from build123d import *

# Parameters (mm, degrees)
SKETCH1_W           = 50
SKETCH1_H           = 40
SKETCH1_R           = 1.5
SKETCH1_R_2         = 0.75
SKETCH1_R_3         = 2.5
BOSS_EXTRUDE1_DEPTH = 2
FILLET1_R           = 0.3
BOSS_EXTRUDE2_START = 1
SKETCH2_R           = 0.65
BOSS_EXTRUDE2_DEPTH = 2.5
FILLET2_R           = 0.1


with BuildPart() as part:
    # Sketch1 → Boss-Extrude1 (new body)
    with BuildSketch(Plane.XY):
        Rectangle(SKETCH1_W, SKETCH1_H)
        with Locations((-23, 18)):
            Circle(SKETCH1_R, mode=Mode.SUBTRACT)
        with Locations((23, -18)):
            Circle(SKETCH1_R, mode=Mode.SUBTRACT)
        with Locations((8, 8)):
            Circle(SKETCH1_R_2, mode=Mode.SUBTRACT)
        with Locations((-8, -8)):
            Circle(SKETCH1_R_2, mode=Mode.SUBTRACT)
        with Locations((-21, -16)):
            Circle(SKETCH1_R_3, mode=Mode.SUBTRACT)
        with Locations((21, 16)):
            Circle(SKETCH1_R_3, mode=Mode.SUBTRACT)
    extrude(amount=BOSS_EXTRUDE1_DEPTH)

    # Fillet1
    fillet1_edges = [part.edges().sort_by_distance(p)[0] for p in [
        (-25, 0, 2),
        (0, -20, 2),
        (25, 0, 2),
        (0, 20, 2),
    ]]
    fillet(fillet1_edges, radius=FILLET1_R)

    # Sketch2 → Boss-Extrude2 (add)
    with BuildSketch(Plane.XY.offset(BOSS_EXTRUDE2_START)):
        with Locations((-8, 8)):
            Circle(SKETCH2_R)
        with Locations((8, -8)):
            Circle(SKETCH2_R)
    extrude(amount=BOSS_EXTRUDE2_DEPTH)

    # Fillet2
    fillet2_edges = [part.edges().sort_by_distance(p)[0] for p in [
        (-8.65, 8, 2),
        (-8.65, 8, 3.5),
        (7.35, -8, 2),
        (7.35, -8, 3.5),
    ]]
    fillet(fillet2_edges, radius=FILLET2_R)


solid = part.part
Geometry: final body of the model. Coordinates: model frame, mm. A direction names the side the tool comes from. Give positions to 0.01 mm unless a question says otherwise; leave off trailing zeros. Loops run counter-clockwise (first coordinate to the right, second up) from the corner with the lowest first, then second, coordinate; pieces in that order, holes last. Notation, with made-up numbers: M 74,86.25 L 94,86.25 A26 ccw 94,111.25 Z; hole C -0.5,42 d8. An arc over 180 degrees is marked long. Put each result on its own line as item: value. Start each with the question number.
1) Cut plane C-C (z = 1.15). Output: boundary loops of the cut face in (x, y).
2) Cut plane A-A (x = 8). Output: boundary loops of the cut face in (y, z).
3) Cut plane B-B (y = -8). Output: boundary loops of the cut face in (x, z).
4) Pull-direction query (Y, two-part tool) for faces 1 (the cylindrical face through (18.5, 16.1, 1)), 2 (the flat face through (0, -20, 1)), 3 (the flat face through (0, 0, 2)); classes: pulls with the +Y half, pulls with the -Y half, needs draft (parallel to the pull), parting line crosses it, or undercut.
5) Access query for faces 4 (the cylindrical face through (7.52, -7.56, 2.74)), 5 (the flat face through (-25, 0, 1)). Directions: +Z, -Z, +X, -X, +Y, -Y. A direction counts if a zero-diameter tool reaches every point of the face in a straight line with its end or side. Return the directions, or none.
6) Ray query, line 1 along Y through (x, z) = (8, 1.15); line 2 along Y through (x, z) = (-23, 1.6); line 3 along Z through (x, y) = (-14, 18). Return the intervals inside material, ascending.
7) Contact query for a flat-ended pin moving along its axis: pin 1 (6 mm diameter, centred on x = -15, y = 4.5, fed in from +Z). Output: stop coordinate, or through.
8) Cut plane D-D (x = -9.5). Output: boundary loops of the cut face in (y, z), then the cut area to 3 significant figures.
Verdict:
1. outline: M -25,-20 L 25,-20 L 25,20 L -25,20 Z; hole C -23,18 d3; hole C -21,-16 d5; hole C -8,-8 d1.5; hole C 8,8 d1.5; hole C 21,16 d5; hole C 23,-18 d3
2. outline: M -20,0 L 7.25,0 L 7.25,2 L -7.25,2 A0.1 cw -7.35,2.1 L -7.35,3.4 A0.1 ccw -7.45,3.5 L -8.55,3.5 A0.1 ccw -8.65,3.4 L -8.65,2.1 A0.1 cw -8.75,2 L -19.7,2 A0.3 ccw -20,1.7 Z; M 8.75,0 L 20,0 L 20,1.7 A0.3 ccw 19.7,2 L 8.75,2 Z
3. outline: M -25,0 L -8.75,0 L -8.75,2 L -24.7,2 A0.3 ccw -25,1.7 Z; M -7.25,0 L 25,0 L 25,1.7 A0.3 ccw 24.7,2 L 8.75,2 A0.1 cw 8.65,2.1 L 8.65,3.4 A0.1 ccw 8.55,3.5 L 7.45,3.5 A0.1 ccw 7.35,3.4 L 7.35,2.1 A0.1 cw 7.25,2 L -7.25,2 Z
4. face 1: undercut
4. face 2: pulls with the -Y half
4. face 3: needs draft
5. face 4: +Z
5. face 5: +Z, -Z, -X, +Y, -Y
6. line 1: -20 to 7.25, 8.75 to 20
6. line 2: -20 to -17.5, -14.5 to 16.5, 19.5 to 20
6. line 3: 0 to 2
7. pin 1: z = 2
8. outline: M -20,0 L 20,0 L 20,1.7 A0.3 ccw 19.7,2 L -19.7,2 A0.3 ccw -20,1.7 Z
8. area: 80.0 mm2
